Verification items for this drawing (mm, ordinates from the low corner). Give positions to 0.01 mm unless a question says otherwise; leave off trailing zeros. Order: outer loops, then holes, each group sorted by start corner. A loop starts at its lowest first (then second) coordinate and runs counter-clockwise, first axis right, second up.
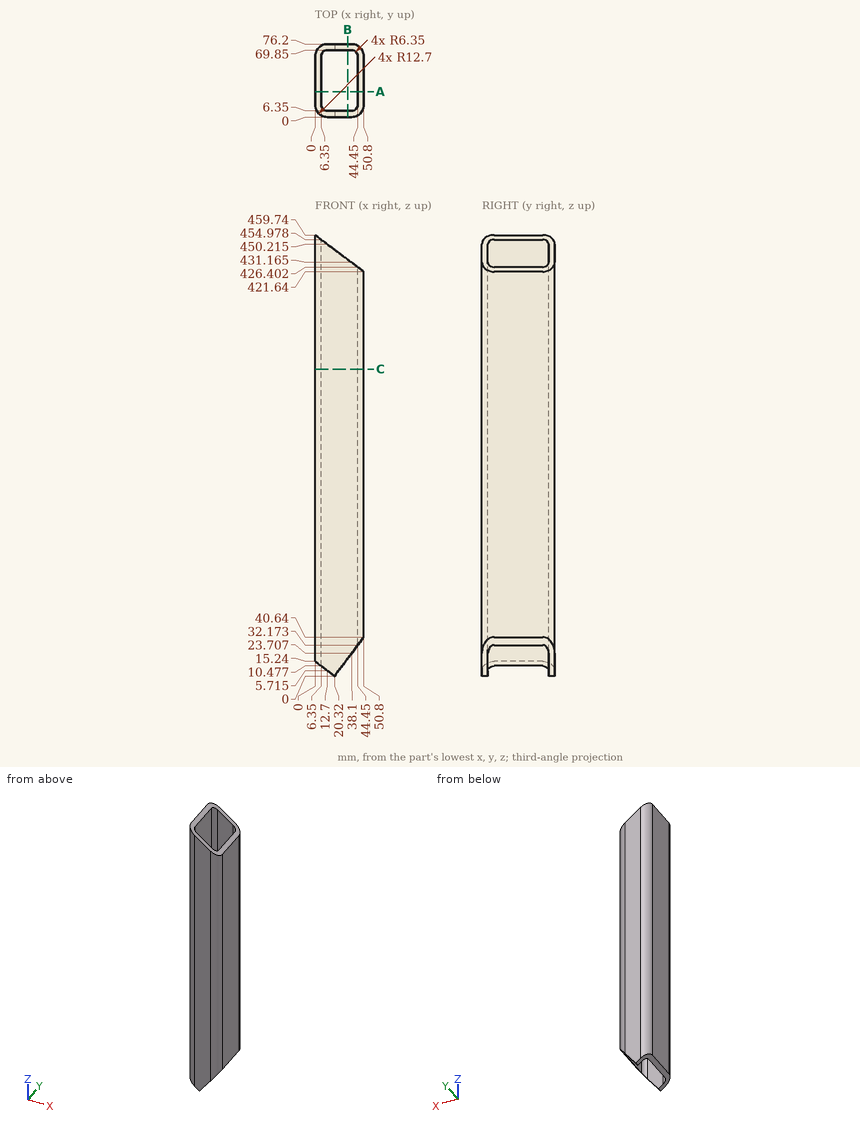
Q1. Cross-section at C-C, the plane z = 320. Record the boundary of the cut face in (x, y), and give its area (3 significant figures).
Q2. Thickness scan on L1, parallel to Y at x = 38, z = 388.5; L2, parallel to X at y = 23, z = 380; L3, parallel to X at y = 64.5, z = 415. Record the ranges inside material, lowest first.
Q3. Cross-section at B-B, the plane x = 34. Record the boundary of the cut face in (y, z), and give its area (3 significant figures).
Q4. Cross-section at A-A, the plane y = 26.5. Record the boundary of the cut face in (x, z).
Q5. Gauge pin test, flat ends, axial feed: P1, Ø8, axis at x = 43, z = 411, coming from the +Y side; P2, Ø1.5, axis at x = 7.5, z = 393.5, coming from the +Y side (1 decimal). Record the tip position at first contact, or that the pin passes through.
Answers follow:
1. outline: (0, 12.7) arc R12.7 ccw to (12.7, 0) - (38.1, 0) arc R12.7 ccw to (50.8, 12.7) - (50.8, 63.5) arc R12.7 ccw to (38.1, 76.2) - (12.7, 76.2) arc R12.7 ccw to (0, 63.5) - close; hole (6.35, 12.7) arc R6.35 ccw to (12.7, 6.35) - (38.1, 6.35) arc R6.35 ccw to (44.45, 12.7) - (44.45, 63.5) arc R6.35 ccw to (38.1, 69.85) - (12.7, 69.85) arc R6.35 ccw to (6.35, 63.5) - close
1. area: 1,350 mm2
2. L1: y = 0 to 6.35, 69.85 to 76.2
2. L2: x = 0 to 6.35, 44.45 to 50.8
2. L3: x = 0.04 to 6.43, 44.37 to 50.76
3. outline: (0, 18.24) - (6.35, 18.24) - (6.35, 434.24) - (0, 434.24) - close; (69.85, 18.24) - (76.2, 18.24) - (76.2, 434.24) - (69.85, 434.24) - close
3. area: 5,280 mm2
4. outline: (0, 15.24) - (6.35, 10.48) - (6.35, 454.98) - (0, 459.74) - close; (44.45, 32.17) - (50.8, 40.64) - (50.8, 421.64) - (44.45, 426.4) - close
5. P1: stops at y = 76.17
5. P2: stops at y = 75.4
